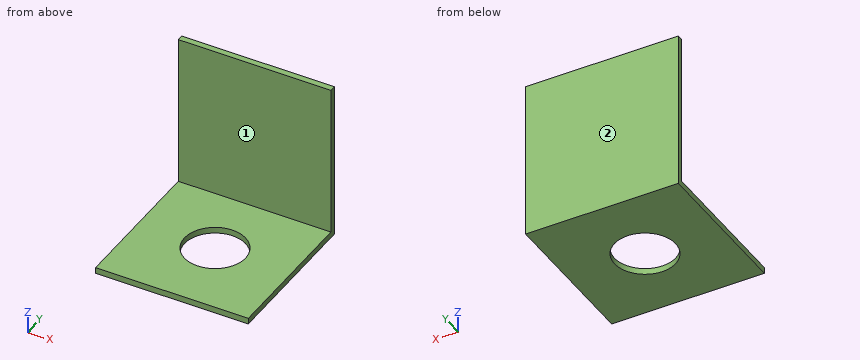
```python
from build123d import *

# Parameters (mm, degrees)
SKETCH1_W           = 50
SKETCH1_H           = 50
BOSS_EXTRUDE1_DEPTH = 2
SKETCH2_W           = 50
SKETCH2_H           = 2
BOSS_EXTRUDE2_DEPTH = 50
SKETCH3_R           = 10
CUT_EXTRUDE2_DEPTH  = 20


with BuildPart() as part:
    # Sketch1 → Boss-Extrude1 (new body)
    with BuildSketch(Plane.XY):
        Rectangle(SKETCH1_W, SKETCH1_H)
    extrude(amount=BOSS_EXTRUDE1_DEPTH)

    # Sketch2 → Boss-Extrude2 (add)
    with BuildSketch(Plane.XY.offset(2)):
        with Locations((0, 24)):
            Rectangle(SKETCH2_W, SKETCH2_H)
    extrude(amount=BOSS_EXTRUDE2_DEPTH)

    # Sketch3 → Cut-Extrude2 (cut)
    with BuildSketch(Plane(origin=(0, 0, 0), x_dir=(-1, 0, 0), z_dir=(0, 0, -1))):
        Circle(SKETCH3_R)
    extrude(amount=-CUT_EXTRUDE2_DEPTH, mode=Mode.SUBTRACT)


solid = part.part
```
The listing builds one solid part. Answer for the finished solid, in the listing's coordinates (mm). Face numbers are marked on the shaded views. A direction names the side the tool comes from. Round coordinates to 2 decimals unless told otherwise and drop trailing zeros. Loops run counter-clockwise (first coordinate to the right, second up) from the corner with the lowest first, then second, coordinate; pieces in that order, holes last. Notation, with made-up numbers: (53.5, 8.5) - (57.5, 8.5) arc R17 ccw to (57.5, 15.5) - close; hole circle Ø11 at (61.25, 20). An arc over 180 degrees is marked (long way). Return JSON: item names as keys, results as strings. Group by question number.
1. The part is cut by section D-D on x = -21. Determine the outline of the cut face in (y, z).
2. Consider probe 1 along Y at (x, z) = (0, 1.2); probe 2 along Y at (x, z) = (19.5, 9); probe 3 along Z at (x, y) = (-20, -1.5). Determine where each line is inside the solid, lowest interval first.
3. The part is cut by section B-B on x = 0. Determine the outline of the cut face in (y, z), then the cut area to 3 significant figures.
4. The part is cut by section C-C on y = 8. Determine the outline of the cut face in (x, z), then the cut area to 3 significant figures.
5. The part is cut by section A-A on y = 0. Determine the outline of the cut face in (x, z), then the cut area to 3 significant figures.
6. Which of the six approach directions +Z, -Z, +X, -X, +Y, -Y give full straight-line access (tool end or side, diameter ignored) to the marked faces 1 and 2?
7. Each of these flat-tipped pins is pushed along its axis until it touches: P1, Ø12, axis at x = 13, z = 7, coming from the -Y side; P2, Ø2, axis at x = -7, z = 18.5, coming from the -Y side; P3, Ø16, axis at x = 0, y = 0, coming from the +Z side. Where does it stop, or does it pass through?
Resolved:
{
 "1": {"outline": "(-25, 0) - (25, 0) - (25, 52) - (23, 52) - (23, 2) - (-25, 2) - close"},
 "2": {"probe 1": "y = -25 to -10, 10 to 25", "probe 2": "y = 23 to 25", "probe 3": "z = 0 to 2"},
 "3": {"outline": "(-25, 0) - (-10, 0) - (-10, 2) - (-25, 2) - close; (10, 0) - (25, 0) - (25, 52) - (23, 52) - (23, 2) - (10, 2) - close", "area": "160 mm²"},
 "4": {"outline": "(-25, 0) - (-6, 0) - (-6, 2) - (-25, 2) - close; (6, 0) - (25, 0) - (25, 2) - (6, 2) - close", "area": "76.0 mm²"},
 "5": {"outline": "(-25, 0) - (-10, 0) - (-10, 2) - (-25, 2) - close; (10, 0) - (25, 0) - (25, 2) - (10, 2) - close", "area": "60.0 mm²"},
 "6": {"face 1": "+Z, +X, -X, -Y", "face 2": "+Z, -Z, +X, -X, +Y"},
 "7": {"P1": "stops at y = -25", "P2": "stops at y = 23", "P3": "passes through"}
}
